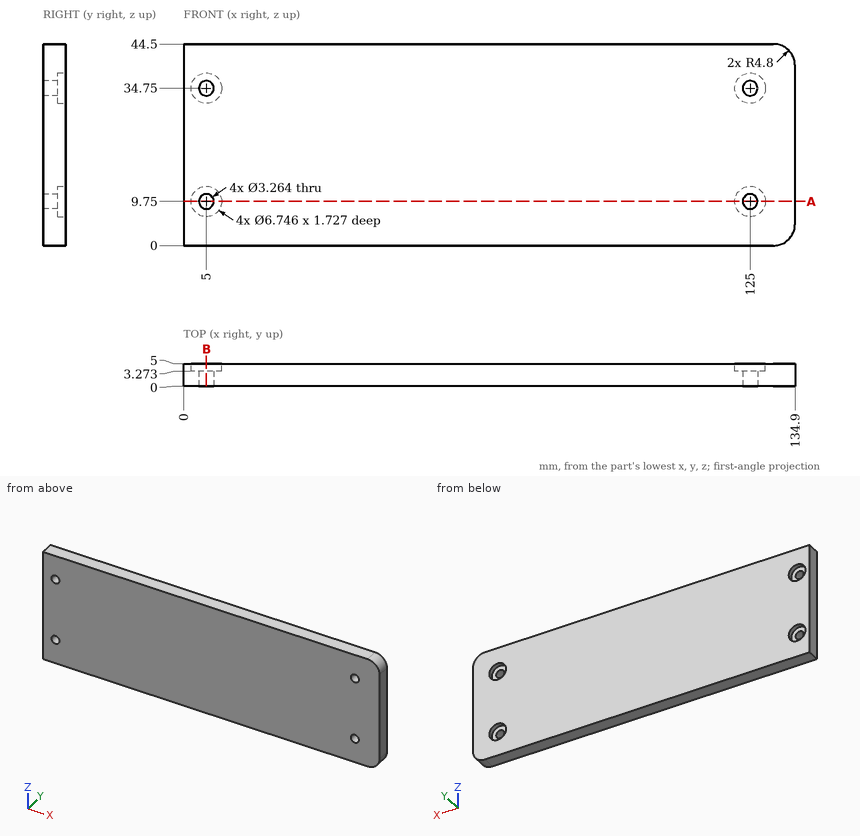
For this review, use the dimensioned drawing (mm, ordinates from the lowest corner) and the shaded views. Round coordinates to 2 decimals unless told otherwise and drop trailing zeros. Order: outer loops, then holes, each group sorted by start corner. A loop starts at its lowest first (then second) coordinate and runs counter-clockwise, first axis right, second up. Notation, with made-up numbers: (-6, 44.5) -> (24, 44.5) arc R20 ccw to (24, 72.5) -> close; hole circle Ø5 at (37.5, 26.5). An arc over 180 degrees is marked (long way). One line per item, written item: value. Start each with the question number.
Q1. Take a section at A-A (z = 9.75). Write out the cut boundary in (x, y).
Q2. Clearance check with flat-ended pins moving along their axes: pin 1 Ø4 at (x, z) = (5, 34.75) entering from -Y; pin 2 Ø3.5 at (x, z) = (4, 35) entering from +Y; pin 3 Ø3 at (x, z) = (125, 34.75) entering from +Y. State where each tip first meets the part, or that it passes through.
Q3. Wall thickness on line 1 (Z direction, x = 5, y = 3.75); line 2 (X direction, y = 1.7, z = 10); line 3 (X direction, y = 4.45, z = 9.75): over which ranges is each line inside the solid? List them lowest first.
Q4. Take a section at B-B (x = 5). Write out the cut boundary in (y, z), and give its area (3 significant figures).
Reported:
1. outline: (0, 0) -> (3.37, 0) -> (3.37, 3.27) -> (1.63, 3.27) -> (1.63, 5) -> (0, 5) -> close; (6.63, 0) -> (123.37, 0) -> (123.37, 3.27) -> (121.63, 3.27) -> (121.63, 5) -> (8.37, 5) -> (8.37, 3.27) -> (6.63, 3.27) -> close; (126.63, 0) -> (134.9, 0) -> (134.9, 5) -> (128.37, 5) -> (128.37, 3.27) -> (126.63, 3.27) -> close
2. pin 1: stops at y = 0
2. pin 2: stops at y = 3.27
2. pin 3: passes through
3. line 1: z = 0 to 6.38, 13.12 to 31.38, 38.12 to 44.5
3. line 2: x = 0 to 3.39, 6.61 to 123.39, 126.61 to 134.9
3. line 3: x = 0 to 1.63, 8.37 to 121.63, 128.37 to 134.9
4. outline: (0, 0) -> (5, 0) -> (5, 6.38) -> (3.27, 6.38) -> (3.27, 8.12) -> (0, 8.12) -> close; (0, 11.38) -> (3.27, 11.38) -> (3.27, 13.12) -> (5, 13.12) -> (5, 31.38) -> (3.27, 31.38) -> (3.27, 33.12) -> (0, 33.12) -> close; (0, 36.38) -> (3.27, 36.38) -> (3.27, 38.12) -> (5, 38.12) -> (5, 44.5) -> (0, 44.5) -> close
4. area: 178 mm2
